```python
from build123d import *

# Parameters (mm, degrees)
BOSS_EXTRUDE1_DEPTH = 20
SKETCH2_R           = 2.5
SKETCH2_W           = 30
SKETCH2_H           = 5
CUT_EXTRUDE1_DEPTH  = 40.05124838


with BuildPart() as part:
    # Sketch1 → Boss-Extrude1 (new, symmetric)
    with BuildSketch(Plane.XY):
        Polygon((0, 0), (15, 0), (15, 30), (10, 30), (0, 15), align=None)
    extrude(amount=BOSS_EXTRUDE1_DEPTH, both=True)

    # Sketch2 → Cut-Extrude1 (cut, through all)
    with BuildSketch(Plane(origin=(15, 0, 0), x_dir=(0, 0, -1), z_dir=(1, 0, 0))):
        with Locations((10, 10)):
            Circle(SKETCH2_R)
        with Locations(Location((-10, 10, 0), (0, 0, 180))):
            Circle(SKETCH2_R)
        with Locations((0, 2.5)):
            Rectangle(SKETCH2_W, SKETCH2_H)
    extrude(amount=-CUT_EXTRUDE1_DEPTH, mode=Mode.SUBTRACT)


solid = part.part
```
Verification items for the finished model (mm, model axes). A direction names the side the tool comes from. Give positions to 0.01 mm unless a question says otherwise; leave off trailing zeros. Order: outer loops, then holes, each group sorted by start corner. A loop starts at its lowest first (then second) coordinate and runs counter-clockwise, first axis right, second up. Notation, with made-up numbers: (-23, -3) -> (21, -3) arc R21 ccw to (21, 2) -> close; hole circle Ø6 at (66, -3). An arc over 180 degrees is marked (long way). One line per item, written item: value.
(1) Scan lines: line 1 along Z through (x, y) = (9, 4); line 2 along Z through (x, y) = (7, 9.5); line 3 along Y through (x, z) = (13.75, -14). Record each from-to range of solid material in increasing order. Write a range as [from, to].
Final values:
line 1: [-20, -15], [15, 20]
line 2: [-20, -12.45], [-7.55, 7.55], [12.45, 20]
line 3: [5, 30]
(2) Draft check along Z on faces 3 (the face through (8, 2, 15)), 4 (the face through (7, 12, -20)), 5 (the face through (5.07, 22.605, 0.28)). Enter one of: pulls with the +Z half, pulls with the -Z half, needs draft (parallel to the pull), parting line crosses it, or undercut.
Final values:
face 3: undercut
face 4: pulls with the -Z half
face 5: needs draft
(3) Sectioned sample at C-C on x = 4. Record the cut outline in (y, z).
Final values:
outline: (0, -20) -> (21, -20) -> (21, 20) -> (0, 20) -> (0, 15) -> (5, 15) -> (5, -15) -> (0, -15) -> close; hole circle Ø5 at (10, -10); hole circle Ø5 at (10, 10)
(4) Sectioned sample at D-D on z = 1.5. Record the cut outline in (x, y), then the cut area to 3 significant figures.
Final values:
outline: (0, 5) -> (15, 5) -> (15, 30) -> (10, 30) -> (0, 15) -> close
area: 300 mm^2
(5) Sectioned sample at A-A on z = 10. Record the cut outline in (x, y).
Final values:
outline: (0, 5) -> (15, 5) -> (15, 7.5) -> (0, 7.5) -> close; (0, 12.5) -> (15, 12.5) -> (15, 30) -> (10, 30) -> (0, 15) -> close
(6) Sectioned sample at B-B on y = 10. Record the cut outline in (x, z).
Final values:
outline: (0, -20) -> (15, -20) -> (15, -12.5) -> (0, -12.5) -> close; (0, -7.5) -> (15, -7.5) -> (15, 7.5) -> (0, 7.5) -> close; (0, 12.5) -> (15, 12.5) -> (15, 20) -> (0, 20) -> close
(7) Gauge pin test, flat ends, axial feed: pin 1 (6 mm diameter, centred on y = 19.5, z = -6.5, fed in from -X); pin 2 (1.5 mm diameter, centred on x = 4, z = 12.5, fed in from +Y) (3 decimals); pin 3 (5 mm diameter, centred on x = 5.5, z = 0.5, fed in from -Y). Record the tip position at first contact, or that the pin passes through.
Final values:
pin 1: x = 1
pin 2: y = 22.125
pin 3: y = 5
(8) Tool access check on faces 1 (the face through (8, 2, -15)), 2 (the face through (7, 0, 18)). Record the directions out of +Z, -Z, +X, -X, +Y, -Y that give a thin tool (end or side, any length) a straight path to the whole face; none if there is none.
Final values:
face 1: +X, -X, -Y
face 2: +Z, -Z, +X, -X, -Y
